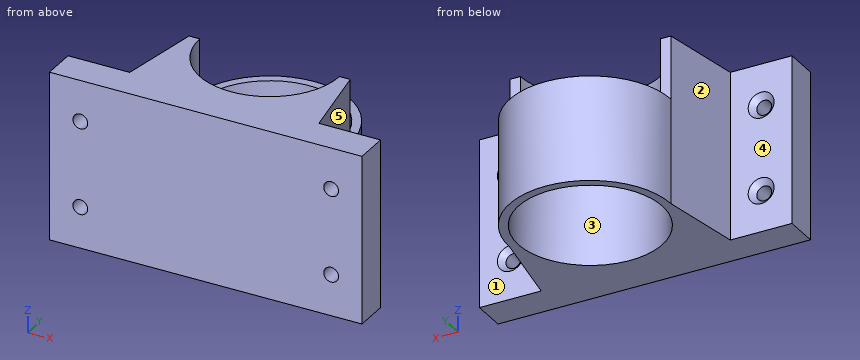
```python
from build123d import *

# Parameters (mm, degrees)
SKETCH1_R                                       = 17.5
BOSS_EXTRUDE9_DEPTH                             = 25.5
BOSS_EXTRUDE10_DEPTH                            = 15.4
BOSS_EXTRUDE10_DEPTH_BACK                       = 25.5
CSK_FOR_M3_FLAT_HEAD_MACHINE_SCREW1_D           = 3.6
CSK_FOR_M3_FLAT_HEAD_MACHINE_SCREW1_CSINK_D     = 6.3
CSK_FOR_M3_FLAT_HEAD_MACHINE_SCREW1_CSINK_ANGLE = 90
CSK_FOR_M3_FLAT_HEAD_MACHINE_SCREW2_D           = 3.6
CSK_FOR_M3_FLAT_HEAD_MACHINE_SCREW2_CSINK_D     = 6.3
CSK_FOR_M3_FLAT_HEAD_MACHINE_SCREW2_CSINK_ANGLE = 90
BOSS_EXTRUDE11_DEPTH                            = 15.4
BOSS_EXTRUDE12_START                            = 3.175
SKETCH15_W                                      = 76
SKETCH15_H                                      = 40.9
SKETCH15_R                                      = 1.8
BOSS_EXTRUDE12_DEPTH                            = 3.175


with BuildPart() as part:
    # Sketch1 → Boss-Extrude9 (new body)
    with BuildSketch(Plane.XY):
        with BuildLine():
            ThreePointArc((-19.6, 18.153395679), (0, 37.753395679), (19.6, 18.153395679))
            ThreePointArc((19.6, 18.153395679), (0, -1.446604321), (-19.6, 18.153395679))
        make_face()
        with Locations((0, 18.153395679)):
            Circle(SKETCH1_R, mode=Mode.SUBTRACT)
    extrude(amount=-BOSS_EXTRUDE9_DEPTH)

    # Sketch1_15 → Boss-Extrude10 (add, two sides: drawn at the far end of the back side and taken through both)
    with BuildSketch(Plane.XY.offset(-BOSS_EXTRUDE10_DEPTH_BACK)):
        with BuildLine():
            Line((-23, -1.846604321), (-38, -1.846604321))
            Line((-38, -1.846604321), (-38, -6.846604321))
            Line((-38, -6.846604321), (38, -6.846604321))
            Line((38, -6.846604321), (38, -1.846604321))
            Line((38, -1.846604321), (23, -1.846604321))
            Line((23, -1.846604321), (19.6, 18.153395679))
            ThreePointArc((19.6, 18.153395679), (0, -1.446604321), (-19.6, 18.153395679))
            Line((-19.6, 18.153395679), (-23, -1.846604321))
        make_face()
    extrude(amount=BOSS_EXTRUDE10_DEPTH + BOSS_EXTRUDE10_DEPTH_BACK)

    # CSK for M3 Flat Head Machine Screw1 (through all)
    with Locations(Plane(origin=(0, -1.846604321, 0), x_dir=(1, 0, 0), z_dir=(0, 1, 0))):
        with Locations((-30.5, 15.5), (-30.5, -5.4)):
            CounterSinkHole(CSK_FOR_M3_FLAT_HEAD_MACHINE_SCREW1_D / 2, CSK_FOR_M3_FLAT_HEAD_MACHINE_SCREW1_CSINK_D / 2, counter_sink_angle=CSK_FOR_M3_FLAT_HEAD_MACHINE_SCREW1_CSINK_ANGLE)

    # CSK for M3 Flat Head Machine Screw2 (through all)
    with Locations(Plane(origin=(0, -1.846604321, 0), x_dir=(1, 0, 0), z_dir=(0, 1, 0))):
        with Locations((30.5, -5.4), (30.5, 15.5)):
            CounterSinkHole(CSK_FOR_M3_FLAT_HEAD_MACHINE_SCREW2_D / 2, CSK_FOR_M3_FLAT_HEAD_MACHINE_SCREW2_CSINK_D / 2, counter_sink_angle=CSK_FOR_M3_FLAT_HEAD_MACHINE_SCREW2_CSINK_ANGLE)

    # Sketch1_19 → Boss-Extrude11 (add)
    with BuildSketch(Plane.XY):
        with BuildLine():
            ThreePointArc((-19.6, 18.153395679), (0, -1.446604321), (19.6, 18.153395679))
            Line((19.6, 18.153395679), (17, 18.153395679))
            ThreePointArc((17, 18.153395679), (0, 1.153395679), (-17, 18.153395679))
            Line((-17, 18.153395679), (-19.6, 18.153395679))
        make_face()
    extrude(amount=BOSS_EXTRUDE11_DEPTH)

    # Sketch15 → Boss-Extrude12 (add)
    with BuildSketch(Plane(origin=(0, -6.846604321, 0), x_dir=(-1, 0, 0), z_dir=(0, -1, 0)).offset(BOSS_EXTRUDE12_START)):
        with Locations((0, 5.05)):
            Rectangle(SKETCH15_W, SKETCH15_H)
        with Locations(Location((-30.5, 15.5, 0), (0, 0, 270))):
            Circle(SKETCH15_R, mode=Mode.SUBTRACT)
        with Locations(Location((30.5, -5.4, 0), (0, 0, 270))):
            Circle(SKETCH15_R, mode=Mode.SUBTRACT)
        with Locations(Location((30.5, 15.5, 0), (0, 0, 270))):
            Circle(SKETCH15_R, mode=Mode.SUBTRACT)
        with Locations(Location((-30.5, -5.4, 0), (0, 0, 270))):
            Circle(SKETCH15_R, mode=Mode.SUBTRACT)
    extrude(amount=-BOSS_EXTRUDE12_DEPTH)


solid = part.part
```
Work out the finished part from the listing and answer in its coordinate system (mm). Face numbers are marked on the shaded views. A direction names the side the tool comes from. Round coordinates to 2 decimals unless told otherwise and drop trailing zeros. Loops run counter-clockwise (first coordinate to the right, second up) from the corner with the lowest first, then second, coordinate; pieces in that order, holes last.
(1) The part is cut by section C-C, the plane z = 5.4. Give the vertices of the cut face in (x, y).
Computed values:
outline: (-38, -10.02) - (-32.3, -10.02) - (-32.3, -3.2) - (-33.65, -1.85) - (-38, -1.85) - close; (-28.7, -10.02) - (28.7, -10.02) - (28.7, -3.2) - (27.35, -1.85) - (23, -1.85) - (19.6, 18.15) - (17, 18.15) arc R17 cw to (-17, 18.15) - (-19.6, 18.15) - (-23, -1.85) - (-27.35, -1.85) - (-28.7, -3.2) - close; (32.3, -10.02) - (38, -10.02) - (38, -1.85) - (33.65, -1.85) - (32.3, -3.2) - close
(2) The part is cut by section A-A, the plane z = -15.5. Give the vertices of the cut face in (x, y), and give its area (3 significant figures).
Computed values:
outline: (-38, -10.02) - (-32.3, -10.02) - (-32.3, -3.2) - (-33.65, -1.85) - (-38, -1.85) - close; (-28.7, -10.02) - (28.7, -10.02) - (28.7, -3.2) - (27.35, -1.85) - (23, -1.85) - (19.6, 18.15) arc R19.6 ccw to (-19.6, 18.15) - (-23, -1.85) - (-27.35, -1.85) - (-28.7, -3.2) - close; (32.3, -10.02) - (38, -10.02) - (38, -1.85) - (33.65, -1.85) - (32.3, -3.2) - close; hole circle Ø35 at (0, 18.15)
area: 1,050 mm2
(3) Each of these flat-tipped pins is pushed along its axis until it touches: P1, Ø1, axis at x = -12, z = -5.5, coming from the +Y side; P2, Ø6, axis at x = 30.5, z = -15.5, coming from the +Y side; P3, Ø6, axis at x = -12.5, z = -9, coming from the +Y side; P4, Ø5, axis at y = 0, z = -4.5, coming from the -X side. Where does it stop, or does it pass through?
Computed values:
P1: stops at y = 34.03
P2: stops at y = -2
P3: stops at y = 35.3
P4: stops at x = -38
(4) The part is cut by section B-B, the plane x = 0. Give the vertices of the cut face in (y, z), and give its area (3 significant figures).
Computed values:
outline: (-10.02, -25.5) - (0.65, -25.5) - (0.65, 0) - (1.15, 0) - (1.15, 15.4) - (-10.02, 15.4) - close; (35.65, -25.5) - (37.75, -25.5) - (37.75, 0) - (35.65, 0) - close
area: 498 mm2
(5) The part is cut by section D-D, the plane y = 29.5. Give the vertices of the cut face in (x, z), and give its area (3 significant figures).
Computed values:
outline: (-15.98, -25.5) - (-13.32, -25.5) - (-13.32, 0) - (-15.98, 0) - close; (13.32, -25.5) - (15.98, -25.5) - (15.98, 0) - (13.32, 0) - close
area: 136 mm2
(6) For the marked faces 4 and 5, determine the directions among +Z, -Z, +X, -X, +Y, -Y from which every point of the face is accessible in a straight line to the end or side of a thin tool.
Computed values:
face 4: +Z, -Z, -X, +Y
face 5: +Z, -Z, +X, +Y
(7) The mould has two halves that part along X. Classify the marked faces 1, 2 and 3: pulls with the +X half, pulls with the -X half, needs draft (parallel to the pull), parting line crosses it, or undercut.
Computed values:
face 1: needs draft
face 2: pulls with the -X half
face 3: undercut
(8) Find the intervals of material crossed by L1, parallel to X at y = -7, z = 5.4; L2, parallel to Z at x = 30.5, y = -8.5; L3, parallel to Z at x = 30, y = -8, in increasing order.
Computed values:
L1: x = -38 to -32.3, -28.7 to 28.7, 32.3 to 38
L2: z = -25.5 to -17.3, -13.7 to 3.6, 7.2 to 15.4
L3: z = -25.5 to -17.23, -13.77 to 3.67, 7.13 to 15.4
